from build123d import *

# Parameters (mm, degrees)
SKETCH2_W            = 118
SKETCH2_H            = 65
BOSS_EXTRUDE2_DEPTH  = 1.5
SKETCH4_W            = 118
SKETCH4_H            = 65
SKETCH4_W_2          = 114
SKETCH4_H_2          = 61
BOSS_EXTRUDE3_DEPTH  = 25
SKETCH6_W            = 14
SKETCH6_H            = 65
BOSS_EXTRUDE4_DEPTH  = 3
FILLET1_R            = 6
FILLET1_OF_MIRROR1_R = 6
FILLET2_R            = 2
FILLET3_R            = 1
SKETCH7_W            = 14
SKETCH7_H            = 11
CUT_EXTRUDE1_DEPTH   = 10


with BuildPart() as part:
    # Sketch2 → Boss-Extrude2 (new body)
    with BuildSketch(Plane.XY):
        Rectangle(SKETCH2_W, SKETCH2_H)
    extrude(amount=BOSS_EXTRUDE2_DEPTH)

    # Sketch4 → Boss-Extrude3 (add)
    with BuildSketch(Plane.XY):
        Rectangle(SKETCH4_W, SKETCH4_H)
        Rectangle(SKETCH4_W_2, SKETCH4_H_2, mode=Mode.SUBTRACT)
    extrude(amount=-BOSS_EXTRUDE3_DEPTH)

    # Sketch6 → Boss-Extrude4 (add)
    with BuildSketch(Plane(origin=(0, 0, -25), x_dir=(-1, 0, 0), z_dir=(0, 0, -1))):
        with Locations((66, 0)):
            Rectangle(SKETCH6_W, SKETCH6_H)
        with BuildLine():
            Line((60, -22.5), (60, 22.5))
            ThreePointArc((60, 22.5), (64.5, 27), (69, 22.5))
            Line((69, 22.5), (69, -22.5))
            ThreePointArc((69, -22.5), (64.5, -27), (60, -22.5))
        make_face(mode=Mode.SUBTRACT)
    boss_extrude4 = extrude(amount=-BOSS_EXTRUDE4_DEPTH)

    # Fillet1
    fillet1_edges = [part.edges().sort_by_distance(p)[0] for p in [
        (-73, -32.5, -23.5),
        (-73, 32.5, -23.5),
    ]]
    fillet(fillet1_edges, radius=FILLET1_R)

    # Mirror1: Boss-Extrude4 across plane
    add(boss_extrude4.mirror(Plane(origin=(0, 0, 0), x_dir=(0, 0, 1), z_dir=(1, 0, 0))))

    # Fillet1 of Mirror1
    fillet1_of_mirror1_edges = [part.edges().sort_by_distance(p)[0] for p in [
        (73, -32.5, -23.5),
        (73, 32.5, -23.5),
    ]]
    fillet(fillet1_of_mirror1_edges, radius=FILLET1_OF_MIRROR1_R)

    # Fillet2
    fillet2_edges = [part.edges().sort_by_distance(p)[0] for p in [
        (-59, 32.5, -10.25),
        (-59, -32.5, -10.25),
        (59, 32.5, -10.25),
        (59, -32.5, -10.25),
    ]]
    fillet(fillet2_edges, radius=FILLET2_R)

    # Fillet3
    fillet3_edges = [part.edges().sort_by_distance(p)[0] for p in [
        (-57, -30.5, -12.5),
        (-57, 30.5, -12.5),
        (57, 30.5, -12.5),
        (57, -30.5, -12.5),
    ]]
    fillet(fillet3_edges, radius=FILLET3_R)

    # Sketch7 → Cut-Extrude1 (cut)
    with BuildSketch(Plane(origin=(59, 0, 0), x_dir=(0, 0, -1), z_dir=(1, 0, 0))):
        with Locations((9.5, -13)):
            Rectangle(SKETCH7_W, SKETCH7_H)
    extrude(amount=-CUT_EXTRUDE1_DEPTH, mode=Mode.SUBTRACT)


solid = part.part
Could you check a few things on this model? Use its own coordinates, in mm. A direction names the side the tool comes from. Give positions to 0.01 mm unless a question says otherwise; leave off trailing zeros. Order: outer loops, then holes, each group sorted by start corner. A loop starts at its lowest first (then second) coordinate and runs counter-clockwise, first axis right, second up. Notation, with made-up numbers: (-13, 87.5) - (21, 87.5) arc R16 cw to (21, 115.5) - close; hole circle Ø1 at (-34, -24). An arc over 180 degrees is marked (long way). One line per question, with ' | ' between items. Start each with the question number.
Item 1: I'm going to push flat-ended pins straight in: pin 1 Ø4 at (y, z) = (12.5, -7) entering from -X; pin 2 Ø5 at (x, y) = (66, 10.5) entering from +Z; pin 3 Ø12.5 at (y, z) = (-2, -8.5) entering from +X; pin 4 Ø1 at (x, z) = (58, -7) entering from +Y. Where does each tip first touch, or does it pass through?
Item 2: Thinking about a two-plate mould opening in X: for faces 1 (the flat face through (-60, 0, -24)), 2 (the flat face through (-73, 0, -24)), 3 (the flat face through (70, 0, -22)), which applies, pulls with the +X half, pulls with the -X half, needs draft (parallel to the pull), parting line crosses it, or undercut?
Item 3: I need wall thicknesses on probe 1 along X at (y, z) = (-17, -23.25); probe 2 along X at (y, z) = (29, -3); probe 3 along Y at (x, z) = (41, -4.75). Which ranges of each line are inside material? Lowest first, please. Write a range as [from, to].
Item 4: I want a section at D-D on x = -64.5. Write out the boundary of the cut face in (y, z).
Item 5: I want a section at C-C on z = -18. Write out the boundary of the cut face in (x, y), then the cut area to 3 significant figures.
Item 6: I want a section at A-A on y = -12. Write out the boundary of the cut face in (x, z), then the cut area to 3 significant figures.
Item 7: I want a section at B-B on x = -19.5. Write out the boundary of the cut face in (y, z), then the cut area to 4 significant figures.
Item 8: For faces 4 (the flat face through (0, -31, -25)), 5 (the flat face through (-59, 0, -10)), 6 (the flat face through (73, 0, -24)), 7 (the cylindrical face through (64.4, 27, -23.5)), 8 (the flat face through (-57, 0, -12)), which set-ups out of +Z, -Z, +X, -X, +Y, -Y let a thin tool reach every point of the face, with its end or its side?
Verdict:
1) pin 1: x = -59 | pin 2: through | pin 3: x = 59 | pin 4: y = 32.44
2) face 1: undercut | face 2: pulls with the -X half | face 3: needs draft
3) probe 1: [-73, -69], [-60, -57], [57, 60], [69, 73] | probe 2: [-59, -57], [57, 59] | probe 3: [-32.5, -30.5], [30.5, 32.5]
4) outline: (-32.5, -25) - (-27, -25) - (-27, -22) - (-32.5, -22) - close; (27, -25) - (32.5, -25) - (32.5, -22) - (27, -22) - close
5) outline: (-59, -30.5) arc R2 ccw to (-57, -32.5) - (57, -32.5) arc R2 ccw to (59, -30.5) - (59, 30.5) arc R2 ccw to (57, 32.5) - (-57, 32.5) arc R2 ccw to (-59, 30.5) - close; hole (-57, -29.5) arc R1 ccw to (-56, -30.5) - (56, -30.5) arc R1 ccw to (57, -29.5) - (57, 29.5) arc R1 ccw to (56, 30.5) - (-56, 30.5) arc R1 ccw to (-57, 29.5) - close | area: 713 mm^2
6) outline: (-73, -25) - (-69, -25) - (-69, -22) - (-73, -22) - close; (-60, -25) - (-57, -25) - (-57, 0) - (57, 0) - (57, -2.5) - (59, -2.5) - (59, 1.5) - (-59, 1.5) - (-59, -22) - (-60, -22) - close; (57, -25) - (60, -25) - (60, -22) - (59, -22) - (59, -16.5) - (57, -16.5) - close; (69, -25) - (73, -25) - (73, -22) - (69, -22) - close | area: 279 mm^2
7) outline: (-32.5, -25) - (-30.5, -25) - (-30.5, 0) - (30.5, 0) - (30.5, -25) - (32.5, -25) - (32.5, 1.5) - (-32.5, 1.5) - close | area: 197.5 mm^2
8) face 4: -Z, +X, -X, +Y, -Y | face 5: +Z, -X, +Y, -Y | face 6: +Z, -Z, +X, +Y, -Y | face 7: +Z, -Z | face 8: -Z
